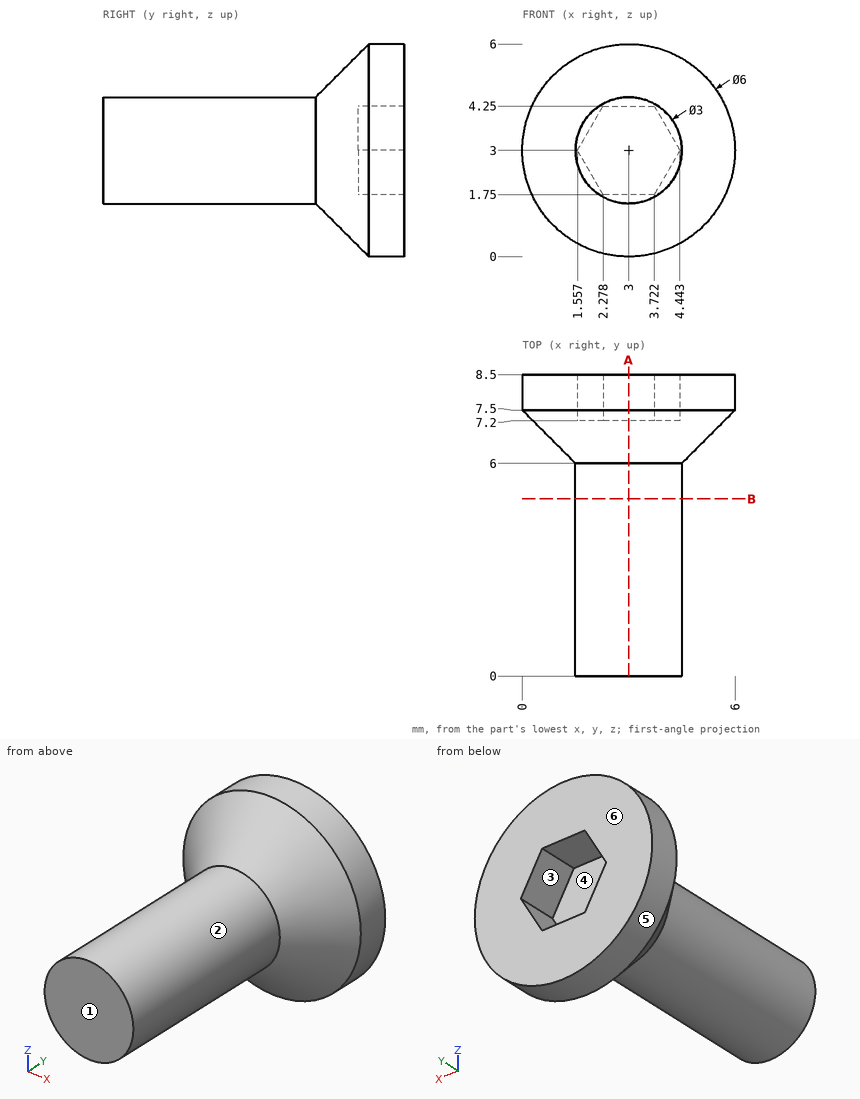
Design review of the part shown in the three views and the two pictorial views. Dimensions are in mm from the part's minimum x, y and z. A direction names the side the tool comes from. Coordinates: 2 decimals unless noted, no trailing zeros. Loops run counter-clockwise (first coordinate to the right, second up) from the corner with the lowest first, then second, coordinate; pieces in that order, holes last. Notation, with made-up numbers: (17, 80) - (29, 80) arc R11 ccw to (29, 95) - close; hole circle Ø9 at (24, 30). An arc over 180 degrees is marked (long way). Use a Markdown table: item, result. Add a question column.
Item 1: For line 1 (Y direction, x = 2.5, z = 3.5); line 2 (X direction, y = 6.5, z = 2); line 3 (Y direction, x = 2.4, z = 0.4), list the stretches that pass through material, from the lowest coordinate up.
Item 2: Insertion check: pin 1 Ø1 at (x, y) = (3, 1.5) entering from -Z; pin 2 Ø2 at (x, z) = (3.5, 3) entering from +Y. Each pin has a flat end and moves straight along its axis. Give the tip position at first contact, or say it passes through.
Item 3: We need section B-B (y = 5). Give the boundary of the cut face in (x, z).
Item 4: Mouldability with a two-part tool opening along X and no side actions: class the marked faces 4, 5 and 6 as pulls with the +X half, pulls with the -X half, needs draft (parallel to the pull), parting line crosses it, or undercut.
Item 5: We need section A-A (x = 3). Give the boundary of the cut face in (y, z).
Item 6: Tool access review of the marked faces 1, 2 and 3: name each direction out of +Z, -Z, +X, -X, +Y, -Y from which nothing blocks a thin tool from reaching the whole face with its end or side.
Results list:
| question | item | result |
|---|---|---|
| 1 | line 1 | y = 0 to 7.2 |
| 1 | line 2 | x = 1.27 to 4.73 |
| 1 | line 3 | y = 7.17 to 8.5 |
| 2 | pin 1 | stops at z = 1.5 |
| 2 | pin 2 | stops at y = 8.5 |
| 3 | outline | circle Ø3 at (3, 3) |
| 4 | face 4 | undercut |
| 4 | face 5 | parting line crosses it |
| 4 | face 6 | needs draft |
| 5 | outline | (0, 1.5) - (6, 1.5) - (7.5, 0) - (8.5, 0) - (8.5, 1.75) - (7.2, 1.75) - (7.2, 4.25) - (8.5, 4.25) - (8.5, 6) - (7.5, 6) - (6, 4.5) - (0, 4.5) - close |
| 6 | face 1 | +Z, -Z, +X, -X, -Y |
| 6 | face 2 | -Y |
| 6 | face 3 | +Y |
